For this review, take the finished solid that the model builds, in its own axes (mm). Round coordinates to 2 decimals unless told otherwise and drop trailing zeros. Loops run counter-clockwise (first coordinate to the right, second up) from the corner with the lowest first, then second, coordinate; pieces in that order, holes last.
```python
from build123d import *

# Parameters (mm, degrees)
SKETCH008_R        = 3
SKETCH012_R        = 3
SKETCH010_R        = 2.75
PAD019_DEPTH       = 14
BODY010_ROLL_ANGLE = 90


with BuildPart() as part:
    # Sketch009 → AdditiveLoft section 0
    with BuildSketch(Plane.XY.offset(14)):
        with BuildLine():
            ThreePointArc((-2.55, 3.55), (-6.1, 0), (-2.55, -3.55))
            Line((-2.55, -3.55), (2.55, -3.55))
            ThreePointArc((2.55, -3.55), (6.1, 0), (2.55, 3.55))
            Line((-2.55, 3.55), (2.55, 3.55))
        make_face()
    # Sketch011 → AdditiveLoft section 1
    with BuildSketch(Plane.XY.offset(14.2)):
        with BuildLine():
            ThreePointArc((-2.55, 3.55), (-6.1, 0), (-2.55, -3.55))
            Line((-2.55, -3.55), (2.55, -3.55))
            ThreePointArc((2.55, -3.55), (6.1, 0), (2.55, 3.55))
            Line((-2.55, 3.55), (2.55, 3.55))
        make_face()
    # Sketch008 → AdditiveLoft section 2
    with BuildSketch(Plane.XY.offset(23.3)):
        Circle(SKETCH008_R)
    # Sketch012 → AdditiveLoft section 3
    with BuildSketch(Plane.XY.offset(23.5)):
        Circle(SKETCH012_R)
    loft()

    # Sketch012 → AdditiveLoft001 section 0
    with BuildSketch(Plane.XY.offset(23.5)):
        Circle(SKETCH012_R)
    # Sketch010 → AdditiveLoft001 section 1
    with BuildSketch(Plane.XY.offset(27.3)):
        Circle(SKETCH010_R)
    loft()

    # Sketch009 → Pad019 (new body)
    with BuildSketch(Plane.XY.offset(14)):
        with BuildLine():
            ThreePointArc((-2.55, 3.55), (-6.1, 0), (-2.55, -3.55))
            Line((-2.55, -3.55), (2.55, -3.55))
            ThreePointArc((2.55, -3.55), (6.1, 0), (2.55, 3.55))
            Line((-2.55, 3.55), (2.55, 3.55))
        make_face()
    extrude(amount=-PAD019_DEPTH)


with BuildPart() as part_1:
    # Body010 roll: moved
    add(part.part.rotate(Axis((0, 0, 0), (1, 0, 0)), BODY010_ROLL_ANGLE))


with BuildPart() as part_2:
    # Body010 placement: moved
    add(part_1.part.moved(Location((0, -6.65, 0))))


solid = part_2.part
```
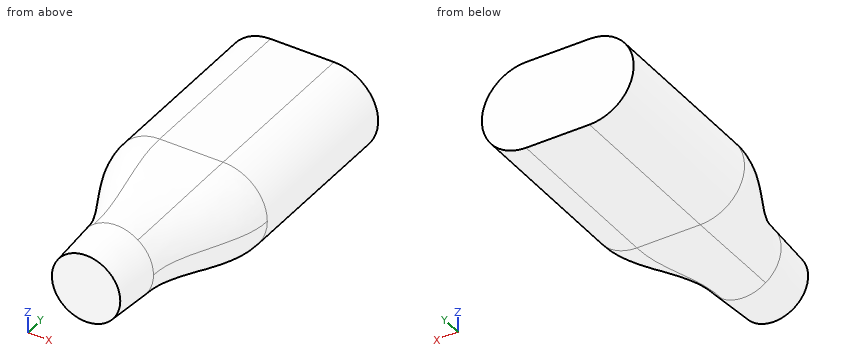
(1) For L1, parallel to Z at x = -4, y = -8; L2, parallel to X at y = -9.5, z = 1.5; L3, parallel to Y at x = -4.5, z = -0.25, list the stretches that pass through material, from the lowest coordinate up.
(2) Insertion check: pin 1 Ø1.5 at (y, z) = (-27, 0) entering from +X; pin 2 Ø2 at (x, y) = (-5, -12.5) entering from -Z; pin 3 Ø1.5 at (x, y) = (-3.5, -30) entering from +Z. Each pin has a flat end and moves straight along its axis. Give the tip position at first contact, or say it passes through.
(3) Add section A-A (y = -11.25). Give the boundary of the cut face in (x, z).
Outcome:
1. L1: z = -3.24 to 3.24
1. L2: x = -5.77 to 5.77
1. L3: y = -25.48 to -6.65
2. pin 1: stops at x = 4.12
2. pin 2: stops at z = -3.24
2. pin 3: stops at z = 1.2
3. outline: (-2.55, -3.55) - (2.55, -3.55) arc R3.55 ccw to (2.55, 3.55) - (-2.55, 3.55) arc R3.55 ccw to start
